Here's how the part is built. I have some questions about the finished solid (model axes, mm). Coordinates: 2 decimals unless noted, no trailing zeros. Write each loop counter-clockwise with the first axis right and the second up, starting at its lowest first coordinate (ties: lowest second). Pieces come first, ordered by that corner, then holes.
Autodesk Inventor part; units mm, degrees
ref_plane "YZ Plane" through (0, 0, 0) normal (1, 0, 0) x (0, 1, 0)
ref_plane "XZ Plane" through (0, 0, 0) normal (0, 1, 0) x (-1, 0, 0)
ref_plane "XY Plane" through (0, 0, 0) normal (0, 0, 1) x (1, 0, 0)
sketch "スケッチ6" plane through (0, 0, 0) normal (0, 0, 1) x (1, 0, 0)
  line L0 (37.5, -17.5) -> (-37.5, -17.5)
  line L1 (-37.5, -17.5) -> (-37.5, 17.5)
  line L2 (-37.5, 17.5) -> (37.5, 17.5)
  line L3 (37.5, 17.5) -> (37.5, -17.5)
  line L4 (37.5, -17.5) -> (-37.5, 17.5) construction
  line L5 (-37.5, -17.5) -> (37.5, 17.5) construction
  point P0 (0, 0)
  dimension "d29" = 75
  dimension "d30" = 35
extrude "押し出し6" add sketch "スケッチ6" along normal blind 3
sketch "スケッチ7" plane through (0, 0, 3) normal (0, 0, 1) x (1, 0, 0)
  circle A0 centre (0, 0) radius 9.75
  dimension "d33" = 19.5
extrude "押し出し7" cut sketch "スケッチ7" against normal blind 3
sketch "スケッチ8" plane through (0, 0, 3) normal (0, 0, 1) x (1, 0, 0)
  circle A0 centre (0, 13) radius 1.65
  circle A1 centre (0, -13) radius 1.65
  circle A2 centre (13, 0) radius 1.65
  circle A3 centre (-13, 0) radius 1.65
  point P0 (0, 0)
  dimension "d36" = 3.3
  dimension "d37" = 3.3
  dimension "d38" = 3.3
  dimension "d39" = 3.3
extrude "押し出し8" cut sketch "スケッチ8" against normal blind 3
sketch "スケッチ9" plane through (0, 0, 3) normal (0, 0, 1) x (1, 0, 0)
  circle A0 centre (-30, 13) radius 2.6
  circle A1 centre (30, 13) radius 2.6
  circle A2 centre (-30, -13) radius 2.6
  circle A3 centre (30, -13) radius 2.6
  point P0 (0, 0)
  dimension "d50" = 5.2
  dimension "d51" = 5.2
  dimension "d52" = 5.2
  dimension "d53" = 5.2
sketch "スケッチ10" plane through (0, 0, 3) normal (0, 0, 1) x (1, 0, 0)
  circle A0 centre (0, 0) radius 16
  dimension "d43" = 32
extrude "押し出し9" cut sketch "スケッチ9" against normal blind 3
fillet "フィレット1" radius 2 4 edges at (-37.5, 17.5, 1.5) (37.5, 17.5, 1.5) (37.5, -17.5, 1.5) (-37.5, -17.5, 1.5)
properties part number "板 中心Φ7" material "アルミニウム 6061"
1) Imagine slicing it at A-A on x = 30. Please give me the cut outline in (y, z), then the cut area to 3 significant figures.
Values follow:
outline: (-17.5, 0) - (-15.6, 0) - (-15.6, 3) - (-17.5, 3) - close; (-10.4, 0) - (10.4, 0) - (10.4, 3) - (-10.4, 3) - close; (15.6, 0) - (17.5, 0) - (17.5, 3) - (15.6, 3) - close
area: 73.8 mm2
2) Imagine slicing it at C-C on x = 0. Please give me the cut outline in (y, z), then the cut area to 3 significant figures.
Values follow:
outline: (-17.5, 0) - (-14.65, 0) - (-14.65, 3) - (-17.5, 3) - close; (-11.35, 0) - (-9.75, 0) - (-9.75, 3) - (-11.35, 3) - close; (9.75, 0) - (11.35, 0) - (11.35, 3) - (9.75, 3) - close; (14.65, 0) - (17.5, 0) - (17.5, 3) - (14.65, 3) - close
area: 26.7 mm2
3) Will these pins go through, and if not, where does the flat tip stop? pin 1 (4.5 mm diameter, centred on x = 30, y = 13, fed in from -Z); pin 2 (6 mm diameter, centred on x = 0.5, y = -9, fed in from -Z).
Values follow:
pin 1: passes through
pin 2: stops at z = 0
4) I need wall thicknesses on probe 1 along Y at (x, z) = (0, 1.15); probe 2 along Y at (x, z) = (-30, 0.9); probe 3 along Y at (x, z) = (1, 2.05). Which ranges of each line are inside material? Lowest first, please.
Values follow:
probe 1: y = -17.5 to -14.65, -11.35 to -9.75, 9.75 to 11.35, 14.65 to 17.5
probe 2: y = -17.5 to -15.6, -10.4 to 10.4, 15.6 to 17.5
probe 3: y = -17.5 to -14.31, -11.69 to -9.7, 9.7 to 11.69, 14.31 to 17.5
5) We'd pull the mould along Y, two halves only. Please class faces 1 (the face through (-32.063, -14.582, 1.521)), 2 (the face through (-0.4, 11.4, 1.5)), 3 (the face through (-9, -8, 0)), 4 (the face through (0, -17.5, 1)): pulls with the +Y half, pulls with the -Y half, needs draft (parallel to the pull), parting line crosses it, or undercut.
Values follow:
face 1: undercut
face 2: undercut
face 3: needs draft
face 4: pulls with the -Y half
6) Imagine slicing it at B-B on y = 13. Please give me the cut outline in (x, z).
Values follow:
outline: (-37.5, 0) - (-32.6, 0) - (-32.6, 3) - (-37.5, 3) - close; (-27.4, 0) - (-1.65, 0) - (-1.65, 3) - (-27.4, 3) - close; (1.65, 0) - (27.4, 0) - (27.4, 3) - (1.65, 3) - close; (32.6, 0) - (37.5, 0) - (37.5, 3) - (32.6, 3) - close
7) Imagine slicing it at D-D on z = 2.1. Count the separate pieces of the cut face and the enclosed holes in it, then the cut area to 3 significant figures.
Values follow:
separate pieces: 1
enclosed holes: 9
area: 2,200 mm2
